Autodesk Inventor part; units mm, degrees
ref_plane "YZ Plane" through (0, 0, 0) normal (1, 0, 0) x (0, 1, 0)
ref_plane "XZ Plane" through (0, 0, 0) normal (0, 1, 0) x (-1, 0, 0)
ref_plane "XY Plane" through (0, 0, 0) normal (0, 0, 1) x (1, 0, 0)
sketch "Sketch1" plane through (0, 0, 0) normal (0, 0, 1) x (1, 0, 0)
  line L0 (-18, 8.1) -> (18, 8.1)
  line L1 (18, 8.1) -> (18, -8.1)
  line L2 (18, -8.1) -> (-18, -8.1)
  line L3 (-18, -8.1) -> (-18, 8.1)
  line L4 (0, 11.34) -> (0, -11.34) construction
  line L5 (-25.2, 0) -> (25.2, 0) construction
  circle A0 centre (0, 0) radius 5
  circle A1 centre (-12, 0) radius 2.55
  circle A2 centre (12, 0) radius 2.55
  dimension "d0" = 16.2
  dimension "d1" = 36
  dimension "d2" = 10
  dimension "d3" = 5.1
  dimension "d4" = 12
  dimension "d5" = 5.1
  dimension "d6" = 12
extrude "Extrusion1" add sketch "Sketch1" along normal blind 10
chamfer "Chamfer1" distance 1 angle 45 2 edges at (-14.55, 0, 10) (9.45, 0, 10)
equation "\"d5\" = d3"
equation "\"d6\" = d4"
properties part number "supporto guide x"
The listing builds one solid part. Answer for the finished solid, in the listing's coordinates (mm). Coordinates: 2 decimals unless noted, no trailing zeros. Write each loop counter-clockwise with the first axis right and the second up, starting at its lowest first coordinate (ties: lowest second). Pieces come first, ordered by that corner, then holes. Notation, with made-up numbers: (25, 26.25) - (70, 26.25) arc R30 ccw to (70, 53.25) - close; hole circle Ø2 at (2.5, 41). An arc over 180 degrees is marked (long way). Return JSON: item names as keys, results as strings. Group by question number.
Q1. The part is cut by section B-B on x = 0. Write down the section's boundary in (y, z).
Q2. For a pull along Y with two mould halves and no side action, classify faces 1 (the cylindrical face through (-14.024, 1.552, 4.437)), 2 (the flat face through (0, 8.1, 5)), 3 (the flat face through (0, -8.1, 5)) as +Y half, -Y half, draft (parallel to the pull), parting line (faces both ways), or undercut.
Q3. The part is cut by section A-A on y = -4. Write down the section's boundary in (x, z).
Q4. Find the intervals of material crossed by line 1 along Y through (x, z) = (12, 5); line 2 along Y through (x, z) = (0, 8); line 3 along X through (y, z) = (-2, 6), in increasing order. Write a range as [from, to].
Q5. The part is cut by section D-D on y = 0. Write down the section's boundary in (x, z), and give its area (3 significant figures).
Q6. The part is cut by section C-C on z = 4. Write down the section's boundary in (x, y).
Evaluation:
{
 "1": {"outline": "(-8.1, 0) - (-5, 0) - (-5, 10) - (-8.1, 10) - close; (5, 0) - (8.1, 0) - (8.1, 10) - (5, 10) - close"},
 "2": {"face 1": "undercut", "face 2": "+Y half", "face 3": "-Y half"},
 "3": {"outline": "(-18, 0) - (-3, 0) - (-3, 10) - (-18, 10) - close; (3, 0) - (18, 0) - (18, 10) - (3, 10) - close"},
 "4": {"line 1": "y = [-8.1, -2.55], [2.55, 8.1]", "line 2": "y = [-8.1, -5], [5, 8.1]", "line 3": "x = [-18, -13.58], [-10.42, -4.58], [4.58, 10.42], [13.58, 18]"},
 "5": {"outline": "(-18, 0) - (-14.55, 0) - (-14.55, 9) - (-15.55, 10) - (-18, 10) - close; (-9.45, 0) - (-5, 0) - (-5, 10) - (-8.45, 10) - (-9.45, 9) - close; (5, 0) - (9.45, 0) - (9.45, 9) - (8.45, 10) - (5, 10) - close; (14.55, 0) - (18, 0) - (18, 10) - (15.55, 10) - (14.55, 9) - close", "area": "156 mm2"},
 "6": {"outline": "(-18, -8.1) - (18, -8.1) - (18, 8.1) - (-18, 8.1) - close; hole circle Ø5.1 at (-12, 0); hole circle Ø10 at (0, 0); hole circle Ø5.1 at (12, 0)"}
}
